Could you check a few things on this drawing? It's one solid part, dimensions in mm from its lowest x, y, z. Give positions to 0.01 mm unless a question says otherwise; leave off trailing zeros. Loops run counter-clockwise (first coordinate to the right, second up) from the corner with the lowest first, then second, coordinate; pieces in that order, holes last. Notation, with made-up numbers: (79, -0.5) - (131, -0.5) arc R17 cw to (131, 31.5) - close; hole circle Ø10 at (26.5, 32). An arc over 180 degrees is marked (long way). Return JSON: item names as keys, results as strings. Group by question number.
(1) If we section it at A-A (x = 3.5): Please give me the cut outline in (y, z), then the cut area to 3 significant figures.
(2) For P1, Ø1.5, axis at x = 14, z = 10, coming from the -Y side; P2, Ø0.8, axis at y = 4, z = 10, coming from the +X side; P3, Ø6, axis at x = 18, z = 4.5, coming from the +Y side, each with a flat end and sliding along its axis, tell me the tip position at first contact or that it passes through.
(3) If we section it at C-C (y = 0.8): Please give me the cut outline in (x, z).
(4) I need wall thicknesses on probe 1 along Y at (x, z) = (21.75, 6.5); probe 2 along X at (y, z) = (0.55, 0.5); probe 3 along X at (y, z) = (3.8, 7). Which ranges of each line are inside material? Lowest first, please. Write a range as [from, to].
(5) If we section it at B-B (z = 9): Please give me the cut outline in (x, y).
(6) If we section it at D-D (z = 2): Please give me the cut outline in (x, y).
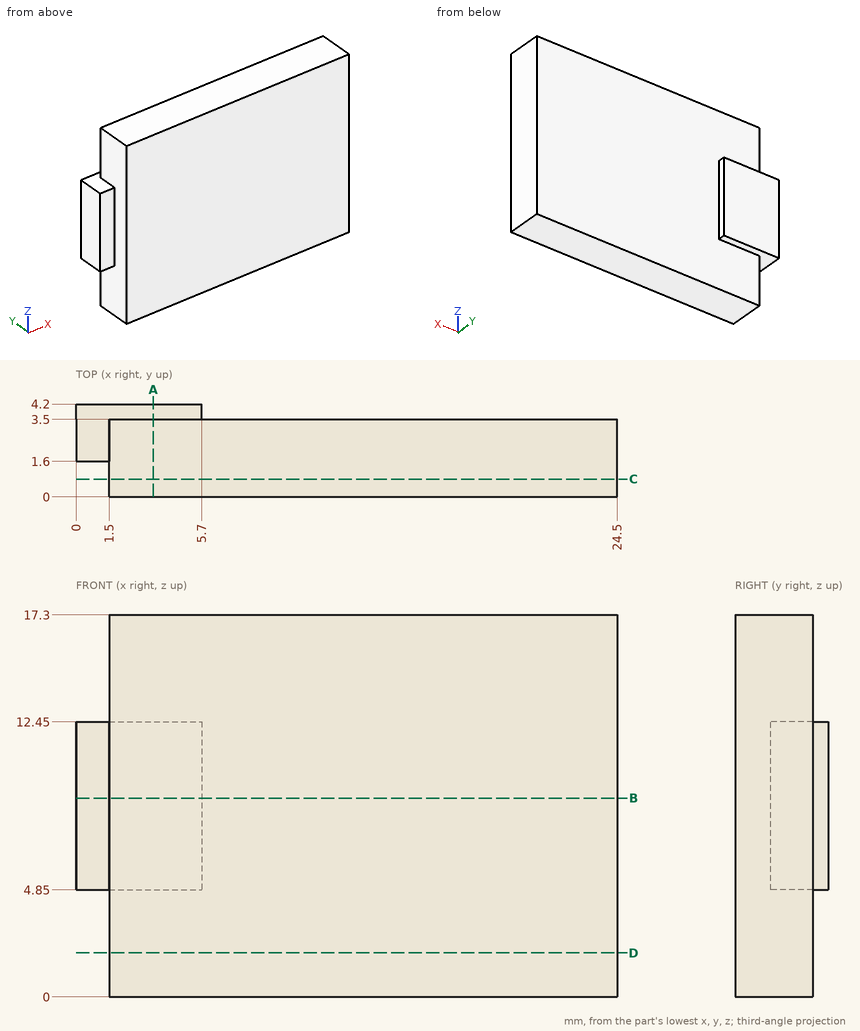
Values:
{
 "1": {"outline": "(0, 0) - (3.5, 0) - (3.5, 4.85) - (4.2, 4.85) - (4.2, 12.45) - (3.5, 12.45) - (3.5, 17.3) - (0, 17.3) - close", "area": "65.9 mm2"},
 "2": {"P1": "y = 0", "P2": "x = 5.7", "P3": "y = 3.5"},
 "3": {"outline": "(1.5, 0) - (24.5, 0) - (24.5, 17.3) - (1.5, 17.3) - close"},
 "4": {"probe 1": "[0, 3.5]", "probe 2": "[1.5, 24.5]", "probe 3": "[0, 5.7]"},
 "5": {"outline": "(0, 1.6) - (1.5, 1.6) - (1.5, 0) - (24.5, 0) - (24.5, 3.5) - (5.7, 3.5) - (5.7, 4.2) - (0, 4.2) - close"},
 "6": {"outline": "(1.5, 0) - (24.5, 0) - (24.5, 3.5) - (1.5, 3.5) - close"}
}
